Read the model definition and answer for the solid it produces. Units are mm, in the model's axes. Round coordinates to 2 decimals unless told otherwise and drop trailing zeros. Order: outer loops, then holes, each group sorted by start corner. A loop starts at its lowest first (then second) coordinate and runs counter-clockwise, first axis right, second up. Notation, with made-up numbers: (75, 23) - (99, 23) arc R29 ccw to (99, 44) - close; hole circle Ø11 at (44.5, 67.25). An arc over 180 degrees is marked (long way). One line per question, with ' | ' between items. Start each with the question number.
1) Straight lines are drawn through the part: line 1 (Y direction, x = 4, z = 1.55); line 2 (X direction, y = 43.98, z = 1.3); line 3 (Y direction, x = -12.45, z = 1.65). For each, find the intervals that lie inside material, in ascending order. Write a range as from..to.
2) The part is cut by section D-D, the plane x = 6. Give the vertices of the cut face in (y, z).
3) A flat-ended cylindrical pin translates along its axis: pin 1 (8 mm diameter, centred on x = -12.45, y = -27.78, fed in from -Z). Find the tip coordinate at first contact, or state that the pin passes through.
4) The part is cut by section A-A, the plane x = -12.45. Give the vertices of the cut face in (y, z).
5) The part is cut by section B-B, the plane y = -47.65. Give the vertices of the cut face in (x, z), plus the area to 3 significant figures.
6) The part is cut by section C-C, the plane z = 1.05. Give the vertices of the cut face in (x, y), plus the area to 3 significant figures.
Autodesk Fusion 360 part; units mm, degrees
sketch "Esboço1" plane through (0, 0, 0) normal (0, 0, 1) x (1, 0, 0)
  line L0 (-20.5, 60) -> (20.5, 60)
  line L1 (22.5, 58) -> (22.5, -58)
  line L2 (20.5, -60) -> (-20.5, -60)
  line L3 (-22.5, -58) -> (-22.5, 58)
  line L4 (-22.5, 60) -> (22.5, -60) construction
  line L5 (22.5, 60) -> (-22.5, -60) construction
  arc A0 (20.5, -60) -> (22.5, -58) centre (20.5, -58) ccw
  arc A1 (22.5, 58) -> (20.5, 60) centre (20.5, 58) ccw
  arc A2 (-20.5, 60) -> (-22.5, 58) centre (-20.5, 58) ccw
  arc A3 (-22.5, -58) -> (-20.5, -60) centre (-20.5, -58) ccw
  dimension "d1" = 45
  dimension "d2" = 120
  dimension "d27" = 2
extrude "Extrusão1" add sketch "Esboço1" along normal blind 2
sketch "Esboço2" plane through (0, 0, 2) normal (0, 0, 1) x (-1, 0, 0)
  line L0 (20.5, 60) -> (-20.5, 60)
  line L1 (-22.5, 58) -> (-22.5, -58)
  line L2 (-20.5, -60) -> (20.5, -60)
  line L3 (22.5, -58) -> (22.5, 58)
  circle A0 centre (12.45, 27.78) radius 2.55
  circle A1 centre (12.45, 47.65) radius 2.55
  line L4 (0.19, -51.5) -> (-13.81, -51.5)
  line L5 (-13.81, -51.5) -> (-13.81, -56.1)
  line L6 (-13.81, -56.1) -> (0.19, -56.1)
  line L7 (0.19, -56.1) -> (0.19, -51.5)
  line L8 (0.19, -51.5) -> (-13.81, -56.1) construction
  line L9 (-13.81, -51.5) -> (0.19, -56.1) construction
  line L10 (-4.26, -44.55) -> (-12.86, -44.55)
  line L11 (-12.86, -44.55) -> (-12.86, -47.55)
  line L12 (-12.86, -47.55) -> (-4.26, -47.55)
  line L13 (-4.26, -47.55) -> (-4.26, -44.55)
  line L14 (-4.26, -44.55) -> (-12.86, -47.55) construction
  line L15 (-12.86, -44.55) -> (-4.26, -47.55) construction
  circle A2 centre (-0.76, -43.98) radius 1.25
  circle A3 centre (-15.86, -43.98) radius 1.25
  arc A4 (20.5, -60) -> (22.5, -58) centre (20.5, -58) ccw
  arc A5 (22.5, 58) -> (20.5, 60) centre (20.5, 58) ccw
  arc A6 (-20.5, 60) -> (-22.5, 58) centre (-20.5, 58) ccw
  arc A7 (-22.5, -58) -> (-20.5, -60) centre (-20.5, -58) ccw
  line L16 (-1.81, -57.3) -> (-11.81, -57.3)
  arc A8 (-11.81, -57.3) -> (-11.81, -58.8) centre (-11.81, -58.05) ccw
  line L17 (-11.81, -58.8) -> (-1.81, -58.8)
  arc A9 (-1.81, -58.8) -> (-1.81, -57.3) centre (-1.81, -58.05) ccw
  line L18 (-1.81, -58.05) -> (-11.81, -58.05) construction
  point P0 (-6.81, -53.8)
  point P1 (-8.56, -46.05)
  dimension "d5" = 5.1
  dimension "d6" = 5.1
  dimension "d7" = 19.87
  dimension "d8" = 10.05
  dimension "d9" = 10.05
  dimension "d11" = 14
  dimension "d12" = 4.6
  dimension "d13" = 8.6
  dimension "d14" = 3
  dimension "d15" = 9.64
  dimension "d16" = 8.69
  dimension "d17" = 3.95
  dimension "d18" = 3.9
  dimension "d19" = 2.5
  dimension "d20" = 2.5
  dimension "d21" = 15.1
  dimension "d22" = 6.64
  dimension "d23" = 16.02
  dimension "d24" = 16.02
  dimension "d29" = 12.35
  dimension "d30" = 1.5
  dimension "d31" = 10
extrude "Extrusão2" cut sketch "Esboço2" against normal blind 15 contours A0 | A1 | L4 L5 L6 L7 | L10 L11 L12 L13 | A2 | A3 | L16 A8 L17 A9
sketch "Esboço4" plane through (0, 0, 2) normal (0, 0, 1) x (-1, 0, 0)
  circle A0 centre (12.45, 27.78) radius 2.55
  circle A1 centre (-15.86, -43.98) radius 1.25
  circle A2 centre (-0.76, -43.98) radius 1.25
  circle A3 centre (12.45, 47.65) radius 2.55
  line L0 (-12.86, -44.55) -> (-4.26, -44.55)
  line L1 (-4.26, -44.55) -> (-4.26, -47.55)
  line L2 (-4.26, -47.55) -> (-12.86, -47.55)
  line L3 (-12.86, -47.55) -> (-12.86, -44.55)
  line L4 (-13.81, -51.5) -> (0.19, -51.5)
  line L5 (0.19, -51.5) -> (0.19, -56.1)
  line L6 (0.19, -56.1) -> (-13.81, -56.1)
  line L7 (-13.81, -56.1) -> (-13.81, -51.5)
  line L8 (-11.81, -57.3) -> (-1.81, -57.3)
  arc A4 (-1.81, -58.8) -> (-1.81, -57.3) centre (-1.81, -58.05) ccw
  line L9 (-1.81, -58.8) -> (-11.81, -58.8)
  arc A5 (-11.81, -57.3) -> (-11.81, -58.8) centre (-11.81, -58.05) ccw
  arc A6 (20.5, -60) -> (22.5, -58) centre (20.5, -58) ccw
  line L10 (22.5, -58) -> (22.5, 58)
  arc A7 (22.5, 58) -> (20.5, 60) centre (20.5, 58) ccw
  line L11 (20.5, 60) -> (-20.5, 60)
  arc A8 (-20.5, 60) -> (-22.5, 58) centre (-20.5, 58) ccw
  line L12 (-22.5, 58) -> (-22.5, -58)
  arc A9 (-22.5, -58) -> (-20.5, -60) centre (-20.5, -58) ccw
  line L13 (-20.5, -60) -> (20.5, -60)
equation "d15 = 5.25 mm + 4.39 mm"
equation "d16 = 4.3 mm + 4.39 mm"
equation "d22 = 2.25 mm + 4.39 mm"
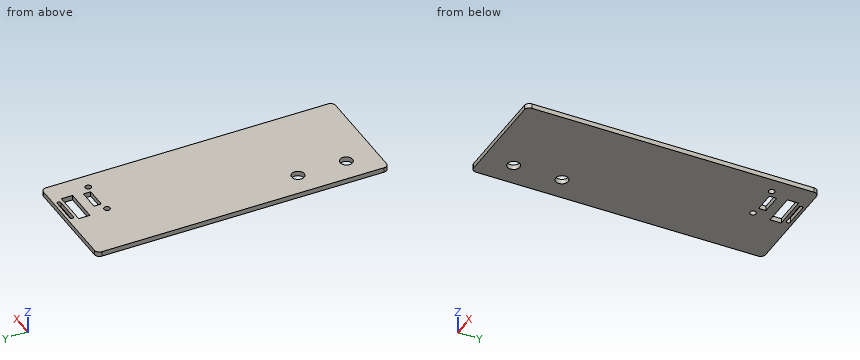
Values:
1) line 1: y = -60..51.5, 56.1..57.3, 58.8..60 | line 2: x = -22.5..-0.49, 2.01..14.61, 17.11..22.5 | line 3: y = -60..-50.2, -45.1..-30.33, -25.23..60
2) outline: (-60, 0) - (44.55, 0) - (44.55, 2) - (-60, 2) - close; (47.55, 0) - (51.5, 0) - (51.5, 2) - (47.55, 2) - close; (56.1, 0) - (57.3, 0) - (57.3, 2) - (56.1, 2) - close; (58.8, 0) - (60, 0) - (60, 2) - (58.8, 2) - close
3) pin 1: stops at z = 0
4) outline: (-60, 0) - (-50.2, 0) - (-50.2, 2) - (-60, 2) - close; (-45.1, 0) - (-30.33, 0) - (-30.33, 2) - (-45.1, 2) - close; (-25.23, 0) - (60, 0) - (60, 2) - (-25.23, 2) - close
5) outline: (-22.5, 0) - (-15, 0) - (-15, 2) - (-22.5, 2) - close; (-9.9, 0) - (22.5, 0) - (22.5, 2) - (-9.9, 2) - close | area: 79.8 mm^2
6) outline: (-22.5, -58) arc R2 ccw to (-20.5, -60) - (20.5, -60) arc R2 ccw to (22.5, -58) - (22.5, 58) arc R2 ccw to (20.5, 60) - (-20.5, 60) arc R2 ccw to (-22.5, 58) - close; hole circle Ø5.1 at (-12.45, -47.65); hole circle Ø5.1 at (-12.45, -27.78); hole circle Ø2.5 at (0.76, 43.98); hole (-0.19, 51.5) - (13.81, 51.5) - (13.81, 56.1) - (-0.19, 56.1) - close; hole (1.81, 57.3) - (11.81, 57.3) arc R0.75 ccw to (11.81, 58.8) - (1.81, 58.8) arc R0.75 ccw to start; hole (4.26, 44.55) - (12.86, 44.55) - (12.86, 47.55) - (4.26, 47.55) - close; hole circle Ø2.5 at (15.86, 43.98) | area: 5,240 mm^2
